Source: CAD feature listing. Evaluate the final solid. Frame: model axes, mm. A direction names the side the tool comes from. Round coordinates to 2 decimals unless told otherwise and drop trailing zeros. Order: outer loops, then holes, each group sorted by start corner. A loop starts at its lowest first (then second) coordinate and runs counter-clockwise, first axis right, second up. Notation, with made-up numbers: (-7, -31) - (51, -31) arc R30 ccw to (51, 4) - close; hole circle Ø3 at (18.25, 65). An arc over 180 degrees is marked (long way). Use one line per item in the form item = value. Start each with the question number.
Q1. Set-up query: faces 4 (the flat face through (103, 70, 22)), 5 (the flat face through (198, 105, 19)), 6 (the flat face through (132, 25, 32)), 7 (the flat face through (187, 120, 19)), 8 (the flat face through (198, 136, 19)). Return all of +Z, -Z, +X, -X, +Y, -Y with unobstructed straight access to the full face (end or side cutting, diameter ignored); none if empty.
Q2. Cut plane C-C, the plane x = 61. Return the cut outline in (y, z).
Q3. Draft query along Y for faces 1 (the flat face through (90, 0, 21)), 2 (the flat face through (89.613, 84.897, 22.325)), 3 (the flat face through (86, 67, 22)). Return one class per face: released by +Y, released by -Y, zero draft, split by the parting line, or undercut.
Q4. Cut plane B-B, the plane y = 20.5. Return the cut outline in (x, z).
Q5. Cut plane D-D, the plane y = 125. Return the cut outline in (x, z), and give its area (3 significant figures).
Q6. Ray query, line 1 (Z direction, x = 21.5, y = 144); line 2 (Y direction, x = 69.5, z = 18); line 3 (Y direction, x = 113, z = 14.5). Return the intervals inside material, ascending. Write a range as [from, to].
Q7. Cut plane A-A, the plane z = 22. Return the cut outline in (x, y).
Q8. Pin query (flat end, axial travel): pin 1 Ø2 at (y, z) = (44, 37.5) entering from +X; pin 2 Ø5 at (x, y) = (143.5, 60) entering from +Z; pin 3 Ø11.5 at (x, y) = (202, 116) entering from +Z. Return the tip coordinate at first contact, or that it passes through.
from build123d import *

# Parameters (mm, degrees)
F0_W     = 235
F0_H     = 155
F1_DEPTH = 10
F2_W     = 107
F2_H     = 50
F3_DEPTH = 45
F4_W     = 23
F4_H     = 31
F5_DEPTH = 18
F7_DEPTH = 25


with BuildPart() as f1:
    # F0 (on Top) → F1 (new body)
    with BuildSketch(Plane.XY):
        with Locations((117.5, 77.5)):
            Rectangle(F0_W, F0_H)
    extrude(amount=F1_DEPTH)

    # F2 (on face) → F3 (join)
    with BuildSketch(Plane.XY.offset(10)):
        with Locations((78.5, 25)):
            Rectangle(F2_W, F2_H)
    extrude(amount=F3_DEPTH)

    # F4 (on face) → F5 (join)
    with BuildSketch(Plane.XY.offset(10)):
        with Locations((198.5, 120.5)):
            Rectangle(F4_W, F4_H)
    extrude(amount=F5_DEPTH)

    # F6 (on face) → F7 (join)
    with BuildSketch(Plane.XY.offset(10)):
        Polygon((100.071068, 95.355339), (78.857864, 74.142136), (93, 60), (114.213203, 81.213203), align=None)
    extrude(amount=F7_DEPTH)


solid = f1.part
Completed:
q1.face_4 = +Z, +X
q1.face_5 = +Z, +X, -X, -Y
q1.face_6 = +Z, +X, +Y, -Y
q1.face_7 = +Z, -X, +Y, -Y
q1.face_8 = +Z, +X, -X, +Y
q2.outline = (0, 0) - (155, 0) - (155, 10) - (50, 10) - (50, 55) - (0, 55) - close
q3.face_1 = released by -Y
q3.face_2 = released by +Y
q3.face_3 = undercut
q4.outline = (0, 0) - (235, 0) - (235, 10) - (132, 10) - (132, 55) - (25, 55) - (25, 10) - (0, 10) - close
q5.outline = (0, 0) - (235, 0) - (235, 10) - (210, 10) - (210, 28) - (187, 28) - (187, 10) - (0, 10) - close
q5.area = 2,760 mm2
q6.line_1 = [0, 10]
q6.line_2 = [0, 50]
q6.line_3 = [0, 50], [80, 82.43]
q7.outline = (25, 0) - (132, 0) - (132, 50) - (25, 50) - close; (78.86, 74.14) - (93, 60) - (114.21, 81.21) - (100.07, 95.36) - close; (187, 105) - (210, 105) - (210, 136) - (187, 136) - close
q8.pin_1 = 132
q8.pin_2 = 10
q8.pin_3 = 28
